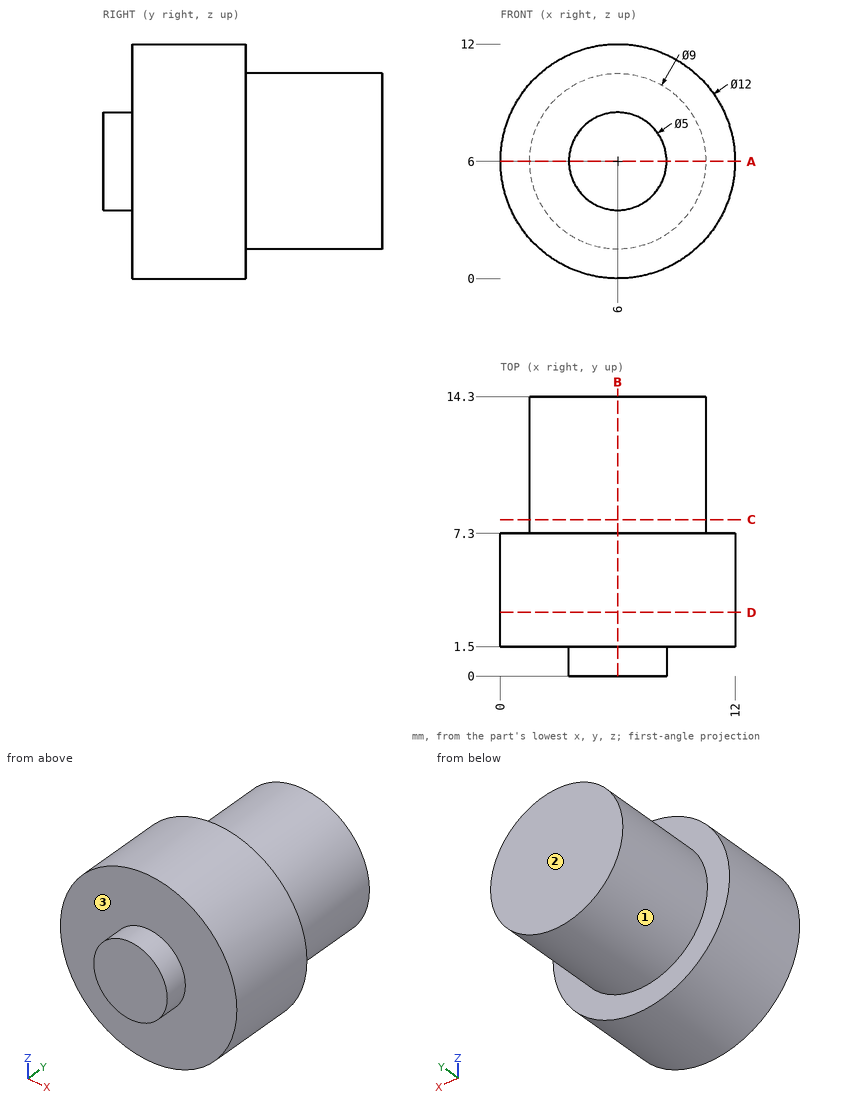
Drawing for the job (mm, zero at the part's lowest x, y, z). A direction names the side the tool comes from. Round coordinates to 2 decimals unless told otherwise and drop trailing zeros. Write each loop counter-clockwise with the first axis right and the second up, starting at its lowest first coordinate (ties: lowest second). Pieces come first, ordered by that corner, then holes. Notation, with made-up numbers: (-19.75, 74) - (12.25, 74) arc R23 cw to (12.25, 94) - close; hole circle Ø4 at (51.5, 5). An arc over 180 degrees is marked (long way). Use CSV: the item, a comma, the result in double quotes.
(1) Pin check, flat tips, straight feed: P1, Ø1, axis at y = 12.5, z = 9.5, coming from the +X side; P2, Ø2, axis at x = 9, y = 10.5, coming from the -Z side; P3, Ø6, axis at x = 4.5, y = 10, coming from the +Z side. Stop position of each tip, or through.
Response:
P1,"x = 9.35"
P2,"z = 1.97"
P3,"z = 12"
(2) Wall check: line 1 (Y direction, x = 6.25, z = 9.5); line 2 (Z direction, x = 6, y = 8); line 3 (Y direction, x = 10.5, z = 2.5). Give the ranges that are in metal, low to high.
Response:
line 1,"1.5 to 14.3"
line 2,"1.5 to 10.5"
line 3,"1.5 to 7.3"
(3) Band-saw the part on D-D (y = 3.25). Write the cut outline in (x, z).
Response:
outline,"circle Ø12 at (6, 6)"
(4) Band-saw the part on B-B (x = 6). Write the cut outline in (y, z).
Response:
outline,"(0, 3.5) - (1.5, 3.5) - (1.5, 0) - (7.3, 0) - (7.3, 1.5) - (14.3, 1.5) - (14.3, 10.5) - (7.3, 10.5) - (7.3, 12) - (1.5, 12) - (1.5, 8.5) - (0, 8.5) - close"
(5) 3-axis set-ups, long thin cutter, end or side, ignore diameter. For the marked faces 1, 2 and 3: which of +Z, -Z, +X, -X, +Y, -Y reach the whole face in a straight line?
Response:
face 1,"+Y"
face 2,"+Z, -Z, +X, -X, +Y"
face 3,"-Y"
(6) Band-saw the part on C-C (y = 8). Write the cut outline in (x, z).
Response:
outline,"circle Ø9 at (6, 6)"
(7) Band-saw the part on A-A (z = 6). Write the cut outline in (x, y), plus the area to 3 significant figures.
Response:
outline,"(0, 1.5) - (3.5, 1.5) - (3.5, 0) - (8.5, 0) - (8.5, 1.5) - (12, 1.5) - (12, 7.3) - (10.5, 7.3) - (10.5, 14.3) - (1.5, 14.3) - (1.5, 7.3) - (0, 7.3) - close"
area,"140 mm²"
